Input: part model. Units: mm. Frame: model coordinates. Face numbers are marked on the shaded views. A direction names the side the tool comes from. Give positions to 0.01 mm unless a question says otherwise; leave off trailing zeros. Write each loop counter-clockwise with the first axis right and the second up, starting at its lowest first coordinate (ties: lowest second). Pieces come first, ordered by that corner, then holes. Notation, with made-up numbers: (3.25, 8.25) -> (24.25, 8.25) arc R16 ccw to (24.25, 31.25) -> close; hole circle Ø2 at (60, 4.5). An arc over 180 degrees is marked (long way). Answer as a JSON object with one key per item and string values. Group by question number.
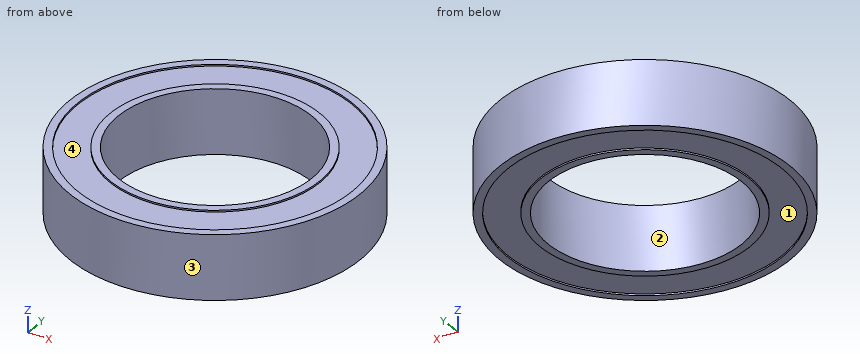
Autodesk Inventor part; units mm, degrees
ref_plane "YZ Plane" through (0, 0, 0) normal (1, 0, 0) x (0, 1, 0)
ref_plane "XZ Plane" through (0, 0, 0) normal (0, 1, 0) x (-1, 0, 0)
ref_plane "XY Plane" through (0, 0, 0) normal (0, 0, 1) x (1, 0, 0)
sketch "Sketch1" plane through (0, 0, 0) normal (1, 0, 0) x (0, 1, 0)
  line L0 (0, 0) -> (0, -2.1848) construction
  line L1 (0, 0) -> (6, 0) construction
  line L2 (6, 0) -> (6, -2)
  line L3 (6, -2) -> (6.5, -2)
  line L4 (6.5, -2) -> (6.5, -1.9)
  line L5 (6.5, -1.9) -> (8.5, -1.9)
  line L6 (8.5, -1.9) -> (8.5, -2)
  line L7 (8.5, -2) -> (9, -2)
  line L8 (9, -2) -> (9, 0)
  line L9 (9, 0) -> (6, 0) construction
  line L10 (6, 0) -> (6, 2)
  line L11 (6, 2) -> (6.5, 2)
  line L12 (6.5, 2) -> (6.5, 1.9)
  line L13 (6.5, 1.9) -> (8.5, 1.9)
  line L14 (8.5, 1.9) -> (8.5, 2)
  line L15 (8.5, 2) -> (9, 2)
  line L16 (9, 2) -> (9, 0)
  dimension "d0" = 6
  dimension "d1" = 9
  dimension "d2" = 0.1
  dimension "d3" = 2
  dimension "d6" = 4
revolve "Revolution1" add sketch "Sketch1" angle 360 about axis through (0, 0, 0) along (0, 0, -1)
properties part number "6701 bearing"
1. Section A-A (x = 0). Return the cut outline in (y, z), plus the area to 3 significant figures.
2. Section C-C (z = 0.7). Return the cut outline in (x, y).
3. Section D-D (y = -7.5). Return the cut outline in (x, z).
4. Line query: line 1 (X direction, y = 0, z = 0.5); line 2 (Y direction, x = 0.25, z = -0.05); line 3 (Z direction, x = 5.5, y = -3.75). Output: solid intervals per line, ascending.
5. Reachability of the marked faces 1 and 2 from +Z, -Z, +X, -X, +Y, -Y: full face, straight path, thin tool, end or side. Return the list, or none.
6. Mould query, pull axis X, two halves, no side actions, for the marked faces 3 and 4. Classes: pulls with the +X half, pulls with the -X half, needs draft (parallel to the pull), parting line crosses it, or undercut.
Working result:
{
 "1": {"outline": "(-9, -2) -> (-8.5, -2) -> (-8.5, -1.9) -> (-6.5, -1.9) -> (-6.5, -2) -> (-6, -2) -> (-6, 2) -> (-6.5, 2) -> (-6.5, 1.9) -> (-8.5, 1.9) -> (-8.5, 2) -> (-9, 2) -> close; (6, -2) -> (6.5, -2) -> (6.5, -1.9) -> (8.5, -1.9) -> (8.5, -2) -> (9, -2) -> (9, 2) -> (8.5, 2) -> (8.5, 1.9) -> (6.5, 1.9) -> (6.5, 2) -> (6, 2) -> close", "area": "23.2 mm^2"},
 "2": {"outline": "circle Ø18 at (0, 0); hole circle Ø12 at (0, 0)"},
 "3": {"outline": "(-4.97, -2) -> (-4, -2) -> (-4, -1.9) -> (4, -1.9) -> (4, -2) -> (4.97, -2) -> (4.97, 2) -> (4, 2) -> (4, 1.9) -> (-4, 1.9) -> (-4, 2) -> (-4.97, 2) -> close"},
 "4": {"line 1": "x = -9 to -6, 6 to 9", "line 2": "y = -9 to -5.99, 5.99 to 9", "line 3": "z = -1.9 to 1.9"},
 "5": {"face 1": "-Z", "face 2": "+Z, -Z"},
 "6": {"face 3": "parting line crosses it", "face 4": "undercut"}
}
